```python
from build123d import *

# Parameters (mm, degrees)
BOSS_EXTRU_1_DEPTH      = 10
ESQUISSE3_R             = 2
ENL_V_MAT_EXTRU_1_DEPTH = 10
CONG_1_R                = 10
ESQUISSE4_R             = 2
ENL_V_MAT_EXTRU_2_DEPTH = 10
ESQUISSE6_R             = 6
ENL_V_MAT_EXTRU_4_DEPTH = 5


with BuildPart() as part:
    # Esquisse2 → Boss.-Extru.1 (new body)
    with BuildSketch(Plane(origin=(0, 0, 0), x_dir=(1, 0, 0), z_dir=(0, 1, 0))):
        with BuildLine():
            Line((0, 0), (290, 0))
            Line((290, 0), (290, 290))
            Line((290, 290), (260, 290))
            ThreePointArc((260, 290), (145, 175), (30, 290))
            Line((30, 290), (0, 290))
            Line((0, 290), (0, 0))
        make_face()
    extrude(amount=BOSS_EXTRU_1_DEPTH)

    # Esquisse3 → Enlèv. mat.-Extru.1 (cut)
    with BuildSketch(Plane(origin=(0, 10, 0), x_dir=(1, 0, 0), z_dir=(0, 1, 0))):
        with Locations((10, 280)):
            Circle(ESQUISSE3_R)
        with Locations((280, 280)):
            Circle(ESQUISSE3_R)
        with Locations((280, 10)):
            Circle(ESQUISSE3_R)
        with Locations((10, 10)):
            Circle(ESQUISSE3_R)
    extrude(amount=-ENL_V_MAT_EXTRU_1_DEPTH, mode=Mode.SUBTRACT)

    # Congé1
    cong_1_edges = [part.edges().sort_by_distance(p)[0] for p in [
        (0, 5, -290),
        (290, 5, -290),
        (290, 5, 0),
        (0, 5, 0),
    ]]
    fillet(cong_1_edges, radius=CONG_1_R)

    # Esquisse4 → Enlèv. mat.-Extru.2 (cut)
    with BuildSketch(Plane(origin=(0, 10, 0), x_dir=(1, 0, 0), z_dir=(0, 1, 0))):
        with Locations((10, 165)):
            Circle(ESQUISSE4_R)
        with Locations((280, 165)):
            Circle(ESQUISSE4_R)
    extrude(amount=-ENL_V_MAT_EXTRU_2_DEPTH, mode=Mode.SUBTRACT)

    # Esquisse6 → Enlèv. mat.-Extru.4 (cut)
    with BuildSketch(Plane.XZ):
        with Locations((10, -10)):
            Circle(ESQUISSE6_R)
        with Locations((280, -10)):
            Circle(ESQUISSE6_R)
        with Locations((280, -165)):
            Circle(ESQUISSE6_R)
        with Locations((280, -280)):
            Circle(ESQUISSE6_R)
        with Locations((10, -280)):
            Circle(ESQUISSE6_R)
        with Locations((10, -165)):
            Circle(ESQUISSE6_R)
    extrude(amount=-ENL_V_MAT_EXTRU_4_DEPTH, mode=Mode.SUBTRACT)


solid = part.part
```
Source: CAD feature listing. Evaluate the final solid. Frame: model axes, mm. A direction names the side the tool comes from. Coordinates: 2 decimals unless noted, no trailing zeros. Loops run counter-clockwise (first coordinate to the right, second up) from the corner with the lowest first, then second, coordinate; pieces in that order, holes last. Notation, with made-up numbers: M 85,27 L 124,27 A14 ccw 124,32 Z; hole C 54,32 d6. An arc over 180 degrees is marked long. Use CSV: the item, a comma, the result in double quotes.
(1) Line query: line 1 (Z direction, x = 10, y = 8.75); line 2 (Z direction, x = 280, y = 1.8); line 3 (X direction, y = 5.25, z = -236). Output: solid intervals per line, ascending. Write a range as [from, to].
Answers follow:
line 1,"[-290, -282], [-278, -167], [-163, -12], [-8, 0]"
line 2,"[-290, -286], [-274, -171], [-159, -16], [-4, 0]"
line 3,"[0, 43.47], [246.53, 290]"
(2) Draft query along X for faces 1 (the face through (8.699, 2.465, -170.857)), 2 (the face through (290, 5, -143)), 3 (the face through (270, 5, -290)). Return one class per face: pulls with the +X half, pulls with the -X half, needs draft (parallel to the pull), parting line crosses it, or undercut.
Answers follow:
face 1,"undercut"
face 2,"pulls with the +X half"
face 3,"needs draft"
(3) Cut plane A-A on z = -238.5. Return loops of the section in (x, y), and give its area (3 significant figures).
Answers follow:
outline,"M 0,0 L 42.18,0 L 42.18,10 L 0,10 Z; M 247.82,0 L 290,0 L 290,10 L 247.82,10 Z"
area,"844 mm²"
(4) Cut plane B-B on y = 8. Return loops of the section in (x, z), and give its area (3 significant figures).
Answers follow:
outline,"M 0,-280 A10 ccw 10,-290 L 30,-290 A115 cw 260,-290 L 280,-290 A10 ccw 290,-280 L 290,-10 A10 ccw 280,0 L 10,0 A10 ccw 0,-10 Z; hole C 10,-280 d4; hole C 10,-165 d4; hole C 10,-10 d4; hole C 280,-280 d4; hole C 280,-165 d4; hole C 280,-10 d4"
area,"63,200 mm²"
(5) Reachability of faces 4 (the face through (280, 5, -168)), 5 (the face through (147.529, 4.93, -175.028)) from +Z, -Z, +X, -X, +Y, -Y: full face, straight path, thin tool, end or side. Return the list, or none.
Answers follow:
face 4,"-Y"
face 5,"-Z, +Y, -Y"
(6) Contact query for flat-ended pins moving along their axis: pin 1 (1.5 mm diameter, centred on x = 176, y = 7.5, fed in from -Z); pin 2 (6 mm diameter, centred on x = 9, z = -165.5, fed in from -Y); pin 3 (2.5 mm diameter, centred on x = 10, z = -280, fed in from -Y). Output: stop coordinate, or through.
Answers follow:
pin 1,"z = -179.47"
pin 2,"y = 5"
pin 3,"through"
(7) Cut plane C-C on x = 145. Return loops of the section in (y, z), and give its area (3 significant figures).
Answers follow:
outline,"M 0,-175 L 10,-175 L 10,0 L 0,0 Z"
area,"1,750 mm²"
